Build history of the part. All positions in model axes, mm. A direction names the side the tool comes from. Give positions to 0.01 mm unless a question says otherwise; leave off trailing zeros. Order: outer loops, then holes, each group sorted by start corner. A loop starts at its lowest first (then second) coordinate and runs counter-clockwise, first axis right, second up. Notation, with made-up numbers: (-12.5, -8) - (16.5, -8) arc R21 ccw to (16.5, 27) - close; hole circle Ø7 at (10, 62.5). An arc over 180 degrees is marked (long way). Use a Markdown table: item, result.
from build123d import *

# Parameters (mm, degrees)
SKETCH6_R           = 5
BOSS_EXTRUDE3_DEPTH = 2.5
SKETCH7_R           = 2.5
BOSS_EXTRUDE4_DEPTH = 10
CUT_EXTRUDE1_START  = -8
CUT_EXTRUDE1_DEPTH  = 8
SKETCH9_R           = 1.500000048
CUT_EXTRUDE2_DEPTH  = 5


with BuildPart() as part:
    # Sketch5 → Revolve1 (revolve)
    with BuildSketch(Plane(origin=(0, 0, 0), x_dir=(0, 0, -1), z_dir=(1, 0, 0)), mode=Mode.PRIVATE) as revolve1_sk:
        Polygon((0, 0), (0, 16.5), (20, 16.5), (20, 13.85), (52.6, 13.85), (52.6, 5), (54.8, 5), (54.8, 1.15), (58.1, 1.15), (58.1, 0), align=None)
    revolve(revolve1_sk.sketch.rotate(Axis((0, 0, 0), (0, 0, 1)), 90), axis=Axis((0, 0, 0), (0, 0, 1)))

    # Sketch6 → Boss-Extrude3 (add)
    with BuildSketch(Plane.XY):
        with Locations((0, 6)):
            Circle(SKETCH6_R)
    extrude(amount=BOSS_EXTRUDE3_DEPTH)

    # Sketch7 → Boss-Extrude4 (add)
    with BuildSketch(Plane.XY.offset(2.5)):
        with Locations((0, 6)):
            Circle(SKETCH7_R)
    extrude(amount=BOSS_EXTRUDE4_DEPTH)

    # Sketch8 → Cut-Extrude1 (cut)
    with BuildSketch(Plane.XY.offset(12.5).offset(CUT_EXTRUDE1_START)):
        with BuildLine():
            Line((-1.999999964, 7.500000048), (1.999999964, 7.500000048))
            ThreePointArc((1.999999964, 7.500000048), (0, 8.5), (-1.999999964, 7.500000048))
        make_face()
    extrude(amount=CUT_EXTRUDE1_DEPTH, mode=Mode.SUBTRACT)

    # Sketch9 → Cut-Extrude2 (cut)
    with BuildSketch(Plane.XY):
        with Locations((0, -13.5)):
            Circle(SKETCH9_R)
        with Locations((-11.691342951, 6.75)):
            Circle(SKETCH9_R)
        with Locations((11.691342951, 6.75)):
            Circle(SKETCH9_R)
    extrude(amount=-CUT_EXTRUDE2_DEPTH, mode=Mode.SUBTRACT)


solid = part.part
1) Slice it at A-A (y = 0). Write the cut outline in (x, z).
Computed:
| item | result |
|---|---|
| outline | (-16.5, -20) - (-13.85, -20) - (-13.85, -52.6) - (-5, -52.6) - (-5, -54.8) - (-1.15, -54.8) - (-1.15, -58.1) - (1.15, -58.1) - (1.15, -54.8) - (5, -54.8) - (5, -52.6) - (13.85, -52.6) - (13.85, -20) - (16.5, -20) - (16.5, 0) - (-16.5, 0) - close |
2) Pin check, flat tips, straight feed: P1, Ø1, axis at y = -5, z = -24, coming from the -X side; P2, Ø3.5, axis at x = -11.69, y = 6.75, coming from the -Z side; P3, Ø2, axis at y = -4.5, z = -1, coming from the -X side. Stop position of each tip, or through.
Computed:
| item | result |
|---|---|
| P1 | stops at x = -13.1 |
| P2 | stops at z = -52.6 |
| P3 | stops at x = -16.12 |
3) Slice it at C-C (z = -7.5). Write the cut outline in (x, y).
Computed:
| item | result |
|---|---|
| outline | circle Ø33 at (0, 0) |
4) Two-plate mould, pull along Y, no slides. Class faces 1 (the flat face through (2, 4, 2.5)), 2 (the flat face through (-12, 7, -5)), 3 (the cylindrical face through (0.91, 0.7, -56.47)), 4 (the flat face through (0, 7.5, 8)): +Y half, -Y half, draft (parallel to the pull), parting line (faces both ways), or undercut.
Computed:
| item | result |
|---|---|
| face 1 | draft |
| face 2 | undercut |
| face 3 | parting line |
| face 4 | +Y half |
5) Wall check: line 1 (Y direction, x = 0, z = -2.65); line 2 (Z direction, x = -8, y = 2); line 3 (X direction, y = -13, z = -2). Give the ranges that are in metal, low to high. Write a range as from..to.
Computed:
| item | result |
|---|---|
| line 1 | y = -16.5..-15, -12..16.5 |
| line 2 | z = -52.6..0 |
| line 3 | x = -10.16..-1.41, 1.41..10.16 |
6) Slice it at D-D (y = 6). Write the cut outline in (x, z).
Computed:
| item | result |
|---|---|
| outline | (-15.37, -20) - (-12.48, -20) - (-12.48, -52.6) - (12.48, -52.6) - (12.48, -20) - (15.37, -20) - (15.37, 0) - (12.99, 0) - (12.99, -5) - (10.39, -5) - (10.39, 0) - (5, 0) - (5, 2.5) - (2.5, 2.5) - (2.5, 12.5) - (-2.5, 12.5) - (-2.5, 2.5) - (-5, 2.5) - (-5, 0) - (-10.39, 0) - (-10.39, -5) - (-12.99, -5) - (-12.99, 0) - (-15.37, 0) - close |
7) Tool access for faces 5 (the cylindrical face through (0.806, -12.235, -2.465)), 6 (the flat face through (0, 0, -58.1)), 7 (the flat face through (-6, 0, -52.6)): list every direction of +Z, -Z, +X, -X, +Y, -Y with a clear straight run to the whole face (end or side of a thin tool).
Computed:
| item | result |
|---|---|
| face 5 | +Z |
| face 6 | -Z, +X, -X, +Y, -Y |
| face 7 | -Z |
